Autodesk Inventor part; units mm, degrees
ref_plane "YZ Plane" through (0, 0, 0) normal (1, 0, 0) x (0, 1, 0)
ref_plane "XZ Plane" through (0, 0, 0) normal (0, 1, 0) x (-1, 0, 0)
ref_plane "XY Plane" through (0, 0, 0) normal (0, 0, 1) x (1, 0, 0)
ref_plane "Work Plane1" through (-2209.9027, -145.7269, 0) normal (0, 0, 1) x (1, 0, 0)
sketch "Sketch1" plane through (-2209.9027, -145.7269, 0) normal (0, 0, 1) x (1, 0, 0)
  line L0 (1984.9027, 125.3224) -> (1984.9027, 70.7269)
  line L1 (1984.9027, 70.7269) -> (2394.9027, 70.7269)
  line L2 (2394.9027, 70.7269) -> (2394.9027, 125.3224)
  line L3 (2394.9027, 125.3224) -> (2409.9027, 125.3224)
  line L4 (2409.9027, 125.3224) -> (2409.9027, 220.7269)
  line L5 (2409.9027, 220.7269) -> (2394.9027, 220.7269)
  line L6 (1969.9027, 220.7269) -> (1969.9027, 125.3224)
  line L7 (1969.9027, 125.3224) -> (1984.9027, 125.3224)
  line L8 (1969.9027, 155.7269) -> (1969.9027, 205.7269)
  line L9 (1969.9027, 205.7269) -> (1964.9027, 205.7269)
  line L10 (1964.9027, 155.7269) -> (1964.9027, 205.7269)
  line L11 (1969.9027, 155.7269) -> (1964.9027, 155.7269)
  line L12 (1969.9027, 85.7269) -> (1969.9027, 135.7269)
  line L13 (1969.9027, 135.7269) -> (1964.9027, 135.7269)
  line L14 (1964.9027, 85.7269) -> (1964.9027, 135.7269)
  line L15 (1969.9027, 85.7269) -> (1964.9027, 85.7269)
  line L16 (1964.9027, 155.7269) -> (1969.9027, 155.7269)
  line L17 (1969.9027, 155.7269) -> (1969.9027, 135.7269)
  line L18 (1969.9027, 135.7269) -> (1964.9027, 135.7269)
  line L19 (1964.9027, 135.7269) -> (1964.9027, 155.7269)
  line L20 (1991.136, 206.6179) -> (1964.9027, 206.6179)
  line L21 (1964.9027, 206.6179) -> (1964.9027, 205.7269)
  line L22 (1964.9027, 205.7269) -> (1991.136, 205.7269)
  line L23 (1991.136, 205.7269) -> (1991.136, 206.6179)
  line L24 (1964.9027, 85.7269) -> (1991.136, 85.7269)
  line L25 (1991.136, 85.7269) -> (1991.136, 70.7269)
  line L26 (1991.136, 70.7269) -> (1964.9027, 70.7269)
  line L27 (1964.9027, 70.7269) -> (1964.9027, 85.7269)
  line L28 (1984.9027, 70.7269) -> (1969.9027, 70.7269)
  line L29 (1969.9027, 70.7269) -> (1969.9027, 125.3224)
  line L30 (1969.9027, 125.3224) -> (1984.9027, 125.3224)
  line L31 (1984.9027, 125.3224) -> (1984.9027, 70.7269)
  line L32 (2414.9027, 155.7269) -> (2414.9027, 205.7269)
  line L33 (2414.9027, 205.7269) -> (2409.9027, 205.7269)
  line L34 (2409.9027, 155.7269) -> (2409.9027, 205.7269)
  line L35 (2414.9027, 155.7269) -> (2409.9027, 155.7269)
  line L36 (2414.9027, 85.7269) -> (2414.9027, 135.7269)
  line L37 (2414.9027, 135.7269) -> (2409.9027, 135.7269)
  line L38 (2409.9027, 85.7269) -> (2409.9027, 135.7269)
  line L39 (2414.9027, 85.7269) -> (2409.9027, 85.7269)
  line L40 (2409.9027, 70.7269) -> (2394.9027, 70.7269)
  line L41 (2394.9027, 70.7269) -> (2394.9027, 125.3224)
  line L42 (2394.9027, 125.3224) -> (2409.9027, 125.3224)
  line L43 (2409.9027, 125.3224) -> (2409.9027, 70.7269)
  line L44 (2259.9027, 220.7269) -> (2238.8976, 199.7218)
  line L45 (2139.9027, 100.7269) -> (2104.5473, 136.0822)
  line L46 (2019.9027, 220.7269) -> (2007.4027, 220.7269)
  line L47 (2178.7935, 132.5467) -> (2175.258, 136.0822)
  line L48 (2104.5473, 136.0822) -> (2101.0118, 132.5467)
  line L49 (2101.0118, 132.5467) -> (2079.7986, 153.7599)
  line L50 (2079.7986, 153.7599) -> (2083.3341, 157.2954)
  line L51 (2083.3341, 157.2954) -> (2062.1209, 178.5086)
  line L52 (2062.1209, 178.5086) -> (2058.5854, 174.9731)
  line L53 (2058.5854, 174.9731) -> (2037.3722, 196.1863)
  line L54 (2037.3722, 196.1863) -> (2040.9077, 199.7218)
  line L55 (2238.8976, 199.7218) -> (2242.4332, 196.1863)
  line L56 (2242.4332, 196.1863) -> (2221.22, 174.9731)
  line L57 (2221.22, 174.9731) -> (2217.6844, 178.5086)
  line L58 (2217.6844, 178.5086) -> (2196.4712, 157.2954)
  line L59 (2196.4712, 157.2954) -> (2200.0068, 153.7599)
  line L60 (2200.0068, 153.7599) -> (2178.7935, 132.5467)
  line L61 (2369.9027, 215.7269) -> (2369.9027, 220.7269)
  line L62 (2369.9027, 220.7269) -> (2349.9027, 220.7269)
  line L63 (2349.9027, 220.7269) -> (2349.9027, 215.7269)
  line L64 (2349.9027, 215.7269) -> (2324.9027, 215.7269)
  line L65 (2324.9027, 215.7269) -> (2324.9027, 220.7269)
  line L66 (2007.4027, 220.7269) -> (2007.4027, 215.7269)
  line L67 (2007.4027, 215.7269) -> (1982.4027, 215.7269)
  line L68 (1982.4027, 215.7269) -> (1982.4027, 220.7269)
  line L69 (2394.9027, 220.7269) -> (2394.9027, 215.7269)
  line L70 (2394.9027, 215.7269) -> (2369.9027, 215.7269)
  line L71 (2324.9027, 220.7269) -> (2259.9027, 220.7269)
  line L72 (2175.258, 136.0822) -> (2139.9027, 100.7269)
  line L73 (2040.9077, 199.7218) -> (2019.9027, 220.7269)
  line L74 (1982.4027, 220.7269) -> (1969.9027, 220.7269)
  point P0 (2209.9027, 145.7269)
  point P1 (1991.136, 21.6179)
  point P2 (1991.136, 6.6179)
  point P3 (1969.9027, 85.7269)
  point P4 (820.3787, 21.6179)
  point P5 (1320.3787, 21.6179)
  point P6 (820.3787, 20.4045)
  point P7 (1984.9027, 70.7269)
  point P8 (1305.3787, -34.1911)
  point P9 (820.3787, 21.6179)
  point P10 (2409.9027, 125.3224)
  point P11 (2394.9027, 70.7269)
  point P12 (1969.9027, 206.6179)
extrude "Extrusion1" add sketch "Sketch1" along normal blind 5 contours L7 L6 L22 L23 L20 L74 L68 L67 L66 L46 L73 L54 L53 L52 L51 L50 L49 L48 L45 L72 L47 L60 L59 L58 L57 L56 L55 L44 L71 L65 L64 L63 L62 L61 L70 L69 L5 L4 L3 L2 L1 L25 L24 L0 | L0 L24 L12 L7 | L24 L25 L1 L0 | L0 L26 L29 L24 | L12 L15 L14 L13 L6 | L11 L10 L9 L6 | L2 L3 L38 L43 L40 | L6 L20 L23 L22 | L4 L37 L36 L39 L38 | L4 L33 L32 L35
sketch "Sketch3" plane through (-2209.9027, -145.7269, 5) normal (0, 0, 1) x (1, 0, 0)
  point P0 (2209.9027, 145.7269)
sketch "Sketch4" plane through (-2209.9027, -145.7269, 5) normal (0, 0, 1) x (1, 0, 0)
  line L0 (2324.9027, 175.7269) -> (2349.9027, 175.7269)
  line L1 (2349.9027, 175.7269) -> (2349.9027, 170.7269)
  line L2 (2349.9027, 170.7269) -> (2324.9027, 170.7269)
  line L3 (2324.9027, 170.7269) -> (2324.9027, 175.7269)
  line L4 (1969.9027, 220.7269) -> (1969.9027, 205.7269)
  line L5 (1969.9027, 155.7269) -> (1969.9027, 135.7269)
  line L6 (1969.9027, 135.7269) -> (1964.9027, 135.7269)
  line L7 (1964.9027, 135.7269) -> (1964.9027, 85.7269)
  line L8 (1969.9027, 70.7269) -> (2409.9027, 70.7269)
  line L9 (2409.9027, 85.7269) -> (2414.9027, 85.7269)
  line L10 (2414.9027, 85.7269) -> (2414.9027, 135.7269)
  line L11 (2414.9027, 135.7269) -> (2409.9027, 135.7269)
  line L12 (2409.9027, 135.7269) -> (2409.9027, 155.7269)
  line L13 (2409.9027, 155.7269) -> (2414.9027, 155.7269)
  line L14 (2414.9027, 155.7269) -> (2414.9027, 205.7269)
  line L15 (2414.9027, 205.7269) -> (2409.9027, 205.7269)
  line L16 (2409.9027, 205.7269) -> (2409.9027, 220.7269)
  line L17 (2409.9027, 220.7269) -> (2394.9027, 220.7269)
  line L18 (2369.9027, 175.7269) -> (2394.9027, 175.7269)
  line L19 (2394.9027, 175.7269) -> (2394.9027, 170.7269)
  line L20 (2394.9027, 170.7269) -> (2369.9027, 170.7269)
  line L21 (2369.9027, 170.7269) -> (2369.9027, 175.7269)
  line L22 (2259.9027, 220.7269) -> (2238.8976, 199.7218)
  line L23 (2139.9027, 100.7269) -> (2104.5473, 136.0822)
  line L24 (2019.9027, 220.7269) -> (2007.4027, 220.7269)
  line L25 (1964.9027, 85.7269) -> (1969.9027, 85.7269)
  line L26 (2409.9027, 70.7269) -> (2409.9027, 85.7269)
  line L27 (1969.9027, 85.7269) -> (1969.9027, 70.7269)
  line L28 (1964.9027, 205.7269) -> (1964.9027, 155.7269)
  line L29 (1964.9027, 155.7269) -> (1969.9027, 155.7269)
  line L30 (2238.8976, 199.7218) -> (2242.4332, 196.1863)
  line L31 (2242.4332, 196.1863) -> (2221.22, 174.9731)
  line L32 (2221.22, 174.9731) -> (2217.6844, 178.5086)
  line L33 (2217.6844, 178.5086) -> (2196.4712, 157.2954)
  line L34 (2196.4712, 157.2954) -> (2200.0068, 153.7599)
  line L35 (2200.0068, 153.7599) -> (2178.7935, 132.5467)
  line L36 (2178.7935, 132.5467) -> (2175.258, 136.0822)
  line L37 (2104.5473, 136.0822) -> (2101.0118, 132.5467)
  line L38 (2101.0118, 132.5467) -> (2079.7986, 153.7599)
  line L39 (2079.7986, 153.7599) -> (2083.3341, 157.2954)
  line L40 (2083.3341, 157.2954) -> (2062.1209, 178.5086)
  line L41 (2062.1209, 178.5086) -> (2058.5854, 174.9731)
  line L42 (2058.5854, 174.9731) -> (2037.3722, 196.1863)
  line L43 (2037.3722, 196.1863) -> (2040.9077, 199.7218)
  line L44 (2394.9027, 220.7269) -> (2394.9027, 215.7269)
  line L45 (2394.9027, 215.7269) -> (2369.9027, 215.7269)
  line L46 (2369.9027, 215.7269) -> (2369.9027, 220.7269)
  line L47 (2369.9027, 220.7269) -> (2349.9027, 220.7269)
  line L48 (2349.9027, 220.7269) -> (2349.9027, 215.7269)
  line L49 (2349.9027, 215.7269) -> (2324.9027, 215.7269)
  line L50 (2324.9027, 215.7269) -> (2324.9027, 220.7269)
  line L51 (2007.4027, 220.7269) -> (2007.4027, 215.7269)
  line L52 (2007.4027, 215.7269) -> (1982.4027, 215.7269)
  line L53 (1982.4027, 215.7269) -> (1982.4027, 220.7269)
  line L54 (2324.9027, 220.7269) -> (2259.9027, 220.7269)
  line L55 (2175.258, 136.0822) -> (2139.9027, 100.7269)
  line L56 (2040.9077, 199.7218) -> (2019.9027, 220.7269)
  line L57 (1982.4027, 220.7269) -> (1969.9027, 220.7269)
  line L58 (1969.9027, 205.7269) -> (1964.9027, 205.7269)
  point P0 (2209.9027, 145.7269)
  dimension "d16" = 25
  dimension "d17" = 5
  dimension "d18" = 100
  dimension "d19" = 25
  dimension "d20" = 5
  dimension "d22" = 15
  dimension "d25" = 20
extrude "Extrusion3" cut sketch "Sketch4" against normal blind 5 contours L0 L1 L2 L3 | L18 L19 L20 L21
sketch "Sketch5" plane through (-2209.9027, -145.7269, 5) normal (0, 0, 1) x (1, 0, 0)
  point P0 (2209.9027, 145.7269)
sketch "Sketch6" plane through (-2209.9027, -145.7269, 5) normal (0, 0, 1) x (1, 0, 0)
  line L0 (2394.9027, 175.7269) -> (2394.9027, 170.7269)
  line L1 (2394.9027, 170.7269) -> (2369.9027, 170.7269)
  line L2 (2369.9027, 170.7269) -> (2369.9027, 175.7269)
  line L3 (2369.9027, 175.7269) -> (2394.9027, 175.7269)
  line L4 (2349.9027, 175.7269) -> (2349.9027, 170.7269)
  line L5 (2349.9027, 170.7269) -> (2324.9027, 170.7269)
  line L6 (2324.9027, 170.7269) -> (2324.9027, 175.7269)
  line L7 (2324.9027, 175.7269) -> (2349.9027, 175.7269)
  line L8 (1964.9027, 85.7269) -> (1969.9027, 85.7269)
  line L9 (1969.9027, 85.7269) -> (1969.9027, 70.7269)
  line L10 (1969.9027, 70.7269) -> (2409.9027, 70.7269)
  line L11 (2409.9027, 70.7269) -> (2409.9027, 85.7269)
  line L12 (2409.9027, 85.7269) -> (2414.9027, 85.7269)
  line L13 (2414.9027, 85.7269) -> (2414.9027, 135.7269)
  line L14 (2414.9027, 135.7269) -> (2409.9027, 135.7269)
  line L15 (2409.9027, 135.7269) -> (2409.9027, 155.7269)
  line L16 (2409.9027, 155.7269) -> (2414.9027, 155.7269)
  line L17 (2414.9027, 155.7269) -> (2414.9027, 205.7269)
  line L18 (2414.9027, 205.7269) -> (2409.9027, 205.7269)
  line L19 (2409.9027, 205.7269) -> (2409.9027, 220.7269)
  line L20 (2409.9027, 220.7269) -> (2394.9027, 220.7269)
  line L21 (2394.9027, 220.7269) -> (2394.9027, 215.7269)
  line L22 (2394.9027, 215.7269) -> (2369.9027, 215.7269)
  line L23 (2369.9027, 215.7269) -> (2369.9027, 220.7269)
  line L24 (2369.9027, 220.7269) -> (2349.9027, 220.7269)
  line L25 (2349.9027, 220.7269) -> (2349.9027, 215.7269)
  line L26 (2349.9027, 215.7269) -> (2324.9027, 215.7269)
  line L27 (2324.9027, 215.7269) -> (2324.9027, 220.7269)
  line L28 (2259.9027, 220.7269) -> (2238.8976, 199.7218)
  line L29 (2238.8976, 199.7218) -> (2242.4332, 196.1863)
  line L30 (2242.4332, 196.1863) -> (2221.22, 174.9731)
  line L31 (2221.22, 174.9731) -> (2217.6844, 178.5086)
  line L32 (2217.6844, 178.5086) -> (2196.4712, 157.2954)
  line L33 (2196.4712, 157.2954) -> (2200.0068, 153.7599)
  line L34 (2200.0068, 153.7599) -> (2178.7935, 132.5467)
  line L35 (2178.7935, 132.5467) -> (2175.258, 136.0822)
  line L36 (2139.9027, 100.7269) -> (2104.5473, 136.0822)
  line L37 (2104.5473, 136.0822) -> (2101.0118, 132.5467)
  line L38 (2101.0118, 132.5467) -> (2079.7986, 153.7599)
  line L39 (2079.7986, 153.7599) -> (2083.3341, 157.2954)
  line L40 (2083.3341, 157.2954) -> (2062.1209, 178.5086)
  line L41 (2062.1209, 178.5086) -> (2058.5854, 174.9731)
  line L42 (2058.5854, 174.9731) -> (2037.3722, 196.1863)
  line L43 (2037.3722, 196.1863) -> (2040.9077, 199.7218)
  line L44 (2019.9027, 220.7269) -> (2007.4027, 220.7269)
  line L45 (2007.4027, 220.7269) -> (2007.4027, 215.7269)
  line L46 (2007.4027, 215.7269) -> (1982.4027, 215.7269)
  line L47 (1982.4027, 215.7269) -> (1982.4027, 220.7269)
  line L48 (1969.9027, 220.7269) -> (1969.9027, 205.7269)
  line L49 (1964.9027, 205.7269) -> (1964.9027, 155.7269)
  line L50 (1964.9027, 155.7269) -> (1969.9027, 155.7269)
  line L51 (1969.9027, 155.7269) -> (1969.9027, 135.7269)
  line L52 (1969.9027, 135.7269) -> (1964.9027, 135.7269)
  line L53 (1964.9027, 135.7269) -> (1964.9027, 85.7269)
  line L54 (2339.9027, 100.7269) -> (2359.9027, 100.7269)
  line L55 (2359.9027, 100.7269) -> (2359.9027, 90.7269)
  line L56 (2359.9027, 90.7269) -> (2339.9027, 90.7269)
  line L57 (2339.9027, 90.7269) -> (2339.9027, 100.7269)
  line L58 (2324.9027, 220.7269) -> (2259.9027, 220.7269)
  line L59 (2175.258, 136.0822) -> (2139.9027, 100.7269)
  line L60 (2040.9077, 199.7218) -> (2019.9027, 220.7269)
  line L61 (1982.4027, 220.7269) -> (1969.9027, 220.7269)
  line L62 (1969.9027, 205.7269) -> (1964.9027, 205.7269)
  point P0 (2209.9027, 145.7269)
  dimension "d26" = 20
  dimension "d27" = 10
  dimension "d28" = 20
  dimension "d29" = 50
extrude "Extrusion4" cut sketch "Sketch6" against normal blind 10 contours L54 L55 L56 L57
equation "\"d19\" = d16"
properties part number "Frontal"
Could you check a few things on this model? Use its own coordinates, in mm. A direction names the side the tool comes from. Give positions to 0.01 mm unless a question says otherwise; leave off trailing zeros. Write each loop counter-clockwise with the first axis right and the second up, starting at its lowest first coordinate (ties: lowest second). Pieces come first, ordered by that corner, then holes. Notation, with made-up numbers: (89.5, -38.5) -> (119.5, -38.5) arc R26 ccw to (119.5, 0.5) -> close; hole circle Ø5 at (78, 25). An arc over 180 degrees is marked (long way). Write each question's results on one line, items separated by ' | '. Start each with the question number.
Q1. Suppose I cut it at D-D, the plane x = -134. List the corners of the cut face in (y, z) for me, and give its area (3 significant figures).
Q2. Suppose I cut it at B-B, the plane y = -4. List the corners of the cut face in (x, z) for me.
Q3. I need wall thicknesses on probe 1 along Y at (x, z) = (140.5, 4.7); probe 2 along Y at (x, z) = (-210.5, 3.95); probe 3 along X at (y, z) = (47.5, 0.8). Which ranges of each line are inside material? Lowest first, please.
Q4. Suppose I cut it at A-A, the plane y = -39.5. List the corners of the cut face in (x, z) for me.
Q5. I'm going to push flat-ended pins straight in: pin 1 Ø5 at (x, y) = (140.5, 45) entering from -Z; pin 2 Ø1.5 at (x, z) = (202.5, 3) entering from +Y; pin 3 Ø2.5 at (y, z) = (-1.5, 3) entering from +X; pin 4 Ø1 at (x, z) = (-57, 3.5) entering from +Y. Where does each tip first touch, or does it pass through?
Q6. Which directions (+Z, -Z, +X, -X, +Y, -Y) give clear straight access to the entire face, cutting with the end or side of a thin tool? Please do faces 1 (the face through (40, 65, 2)), 2 (the face through (-23, -16, 0)), 3 (the face through (22.07, 40, 2.46)).
Q7. Suppose I cut it at C-C, the plane z = 3.35. State how many separate pieces and enclosed holes the cut face has, and give its area (3 significant figures).
Q8. We'd pull the mould along X, two halves only. Please class faces 4 (the face through (-23, -16, 5)), 5 (the face through (-137, 22, 2)): +X half, -X half, draft (parallel to the pull), parting line (faces both ways), or undercut.
Outcome:
1) outline: (-75, 0) -> (19, 0) -> (19, 5) -> (-75, 5) -> close | area: 470 mm2
2) outline: (-240, 0) -> (-118.07, 0) -> (-118.07, 5) -> (-240, 5) -> close; (-21.93, 0) -> (200, 0) -> (200, 5) -> (-21.93, 5) -> close
3) probe 1: -75 to -55, -45 to 75 | probe 2: -75 to 70 | probe 3: -245 to -169.57, 29.57 to 205
4) outline: (-245, 0) -> (-75.5, 0) -> (-75.5, 5) -> (-245, 5) -> close; (-64.5, 0) -> (205, 0) -> (205, 5) -> (-64.5, 5) -> close
5) pin 1: z = 0 | pin 2: y = 60 | pin 3: x = 200 | pin 4: y = -31.5
6) face 1: +Z, -Z, +Y | face 2: -Z, +X, -X, +Y, -Y | face 3: +Z, -Z
7) separate pieces: 1 | enclosed holes: 3 | area: 51,200 mm2
8) face 4: draft | face 5: undercut
